from build123d import *

# Parameters (mm, degrees)
CROQUIS1_R              = 18.4
SALIENTE_EXTRUIR1_DEPTH = 21.5
CROQUIS3_R              = 6
SALIENTE_EXTRUIR2_DEPTH = 6
SALIENTE_EXTRUIR3_DEPTH = 16
SALIENTE_EXTRUIR4_DEPTH = 4
CORTAR_EXTRUIR1_DEPTH   = 1
REDONDEO4_R             = 0.4
CROQUIS7_R              = 1.5
CORTAR_EXTRUIR2_DEPTH   = 3


with BuildPart() as part:
    # Croquis1 → Saliente-Extruir1 (new body)
    with BuildSketch(Plane.XY):
        Circle(CROQUIS1_R)
    extrude(amount=SALIENTE_EXTRUIR1_DEPTH)

    # Croquis3 → Saliente-Extruir2 (add)
    with BuildSketch(Plane.XY.offset(21.5)):
        with Locations((0, -7)):
            Circle(CROQUIS3_R)
    extrude(amount=SALIENTE_EXTRUIR2_DEPTH)

    # Croquis4 → Saliente-Extruir3 (add)
    with BuildSketch(Plane.XY.offset(27.5)):
        with BuildLine():
            Line((1.8, -4.6), (-1.8, -4.6))
            ThreePointArc((-1.8, -4.6), (0, -10), (1.8, -4.6))
        make_face()
    extrude(amount=SALIENTE_EXTRUIR3_DEPTH)

    # Croquis5 → Saliente-Extruir4 (add)
    with BuildSketch(Plane.XY.offset(27.5)):
        with BuildLine():
            Line((-1.8, -4.6), (1.8, -4.6))
            ThreePointArc((1.8, -4.6), (0, -4), (-1.8, -4.6))
        make_face()
    extrude(amount=SALIENTE_EXTRUIR4_DEPTH)

    # Croquis6 → Cortar-Extruir1 (cut)
    with BuildSketch(Plane.XY.offset(21.5)):
        with BuildLine():
            ThreePointArc((8.558025235, -9.785714286), (0, 13), (-8.558025235, -9.785714286))
            ThreePointArc((-8.558025235, -9.785714286), (0, 2), (8.558025235, -9.785714286))
        make_face()
    extrude(amount=-CORTAR_EXTRUIR1_DEPTH, mode=Mode.SUBTRACT)

    # Redondeo4
    redondeo4_edges = [part.edges().sort_by_distance(p)[0] for p in [
        (0, 2, 20.5),
        (0, 13, 20.5),
    ]]
    fillet(redondeo4_edges, radius=REDONDEO4_R)

    # Croquis7 → Cortar-Extruir2 (cut)
    with BuildSketch(Plane.XY.offset(21.5)):
        with Locations((-15.4999946, 0)):
            Circle(CROQUIS7_R)
        with Locations((-7.7499973, 13.423389082)):
            Circle(CROQUIS7_R)
        with Locations((7.7499973, 13.423389082)):
            Circle(CROQUIS7_R)
        with Locations((15.4999946, 0)):
            Circle(CROQUIS7_R)
        with Locations((7.7499973, -13.423389082)):
            Circle(CROQUIS7_R)
        with Locations((-7.7499973, -13.423389082)):
            Circle(CROQUIS7_R)
    extrude(amount=-CORTAR_EXTRUIR2_DEPTH, mode=Mode.SUBTRACT)


solid = part.part
Design review of the part built by this model. Coordinates are the model's own, in mm. A direction names the side the tool comes from. Round coordinates to 2 decimals unless told otherwise and drop trailing zeros. Write each loop counter-clockwise with the first axis right and the second up, starting at its lowest first coordinate (ties: lowest second). Pieces come first, ordered by that corner, then holes. Notation, with made-up numbers: (18.25, 13) - (31.25, 13) arc R21 cw to (31.25, 20) - close; hole circle Ø1 at (31.25, 85). An arc over 180 degrees is marked (long way). Return JSON: item names as keys, results as strings. Group by question number.
Item 1: We need section B-B on z = 15.5. Write out the cut boundary in (x, y), and give its area (3 significant figures).
Item 2: Insertion check: P1, Ø1, axis at y = -9, z = 25.5, coming from the -X side; P2, Ø6, axis at x = -4, y = 10, coming from the -Z side; P3, Ø4, axis at x = -7.75, y = -13.42, coming from the +Z side; P4, Ø6, axis at x = -7, z = 10.5, coming from the -Y side. Each pin has a flat end and moves straight along its axis. Give the tip position at first contact, or say it passes through.
Item 3: We need section C-C on z = 34. Write out the cut boundary in (x, y), and give its area (3 significant figures).
Item 4: We need section A-A on x = 0. Write out the cut boundary in (y, z).
Item 5: Machinability: for faces 1 (the face through (-14.6, -11.2, 10.6)), 2 (the face through (-8.08, 11.96, 20.02)), which of the approach directions +Z, -Z, +X, -X, +Y, -Y give a long, thin tool a straight path to every point of the face, cutting with its end or side? Answer none if there is none.
Item 6: For probe 1 along Y at (x, z) = (8.5, 19.5); probe 2 along Z at (x, y) = (-7, 13.5); probe 3 along Z at (x, y) = (4, 2), list the stretches that pass through material, from the lowest coordinate up. Write a range as [from, to].
Item 7: The part is to be moulded in two halves that separate along X. For faces 3 (the face through (0, -7, 43.5)), 4 (the face through (-6, -7, 24)), 5 (the face through (8, 13, 18.5)), 6 (the face through (0.441, 12.993, 21.204)), say which applies: pulls with the +X half, pulls with the -X half, needs draft (parallel to the pull), parting line crosses it, or undercut.
Model answer:
{
 "1": {"outline": "circle Ø36.8 at (0, 0)", "area": "1,060 mm²"},
 "2": {"P1": "stops at x = -5.81", "P2": "stops at z = 0", "P3": "stops at z = 21.5", "P4": "stops at y = -17.96"},
 "3": {"outline": "(-1.8, -4.6) arc R3 ccw (long way) to (1.8, -4.6) - close", "area": "26.8 mm²"},
 "4": {"outline": "(-18.4, 0) - (18.4, 0) - (18.4, 21.5) - (13, 21.5) - (13, 20.9) arc R0.4 cw to (12.6, 20.5) - (2.4, 20.5) arc R0.4 cw to (2, 20.9) - (2, 21.5) - (-1, 21.5) - (-1, 27.5) - (-4, 27.5) - (-4, 31.5) - (-4.6, 31.5) - (-4.6, 43.5) - (-10, 43.5) - (-10, 27.5) - (-13, 27.5) - (-13, 21.5) - (-18.4, 21.5) - close"},
 "5": {"face 1": "+Z, -Z", "face 2": "+Z"},
 "6": {"probe 1": "y = [-16.32, -14.72], [-12.12, 12.12], [14.72, 16.32]", "probe 2": "z = [0, 18.5]", "probe 3": "z = [0, 20.5]"},
 "7": {"face 3": "needs draft", "face 4": "parting line crosses it", "face 5": "undercut", "face 6": "undercut"}
}
